```python
from build123d import *

# Parameters (mm, degrees)
EXTRUDE_THIN1_DEPTH = 10
FILLET1_R           = 5
FILLET2_R           = 5
FILLET3_R           = 5
FILLET4_R           = 5
FILLET5_R           = 5
CUT_EXTRUDE1_DEPTH  = 4.5


with BuildPart() as part:
    # Sketch1 → Extrude-Thin1 (new body)
    with BuildSketch(Plane.XY):
        with BuildLine():
            Line((5, 0), (5, 44.72135955))
            ThreePointArc((5, 44.72135955), (32.200514423, 31.434485377), (44.828761414, 3.922008424))
            Line((44.828761414, 3.922008424), (54.790708395, 4.793565851))
            ThreePointArc((54.790708395, 4.793565851), (35.273871656, 42.198980774), (-5, 54.772255751))
            Line((-5, 54.772255751), (-5, 0))
            Line((-5, 0), (5, 0))
        make_face()
    extrude(amount=EXTRUDE_THIN1_DEPTH)

    # Fillet1
    fillet1_edges = [part.edges().sort_by_distance(p)[0] for p in [
        (-5, 54.772255751, 5),
    ]]
    fillet(fillet1_edges, radius=FILLET1_R)

    # Fillet2
    fillet2_edges = [part.edges().sort_by_distance(p)[0] for p in [
        (54.790708395, 4.793565851, 5),
    ]]
    fillet(fillet2_edges, radius=FILLET2_R)

    # Fillet3
    fillet3_edges = [part.edges().sort_by_distance(p)[0] for p in [
        (44.828761414, 3.922008424, 5),
    ]]
    fillet(fillet3_edges, radius=FILLET3_R - 0.0001)  # a hair under: the kernel refuses the full size

    # Fillet4
    fillet4_edges = [part.edges().sort_by_distance(p)[0] for p in [
        (5, 0, 5),
    ]]
    fillet(fillet4_edges, radius=FILLET4_R)

    # Fillet5
    fillet5_edges = [part.edges().sort_by_distance(p)[0] for p in [
        (-5, 0, 5),
    ]]
    fillet(fillet5_edges, radius=FILLET5_R - 0.0001)  # a hair under: the kernel refuses the full size

    # Sketch2 → Cut-Extrude1 (cut)
    with BuildSketch(Plane(origin=(0, 0, 0), x_dir=(-1, 0, 0), z_dir=(0, 0, -1))):
        with BuildLine():
            Line((1.923996328, 19.347205988), (2.921, 7.13741415))
            ThreePointArc((2.921, 7.13741415), (0, 1.3805), (-2.921, 7.13741415))
            Line((-2.921, 7.13741415), (-1.923996328, 19.347205988))
            ThreePointArc((-1.923996328, 19.347205988), (0, 21.1205), (1.923996328, 19.347205988))
        make_face()
    extrude(amount=-CUT_EXTRUDE1_DEPTH, mode=Mode.SUBTRACT)


solid = part.part
```
Could you check a few things on this model? Use its own coordinates, in mm. A direction names the side the tool comes from. Round coordinates to 2 decimals unless told otherwise and drop trailing zeros. Write each loop counter-clockwise with the first axis right and the second up, starting at its lowest first coordinate (ties: lowest second). Pieces come first, ordered by that corner, then holes. Notation, with made-up numbers: M 41,62 L 54,62 A26 ccw 54,91 Z; hole C 11.5,73 d8. An arc over 180 degrees is marked long. Answer in a Markdown table with one row per item. Add a question column.
Q1. Imagine slicing it at B-B (y = 31.5). Please give me the cut outline in (x, z).
Q2. If we mould it in two halves opening along Y, with no side actions, what happens to faces 1 (the flat face through (-5, 28, 5)), 2 (the cylindrical face through (46.15, 5.3, 5.07)), 3 (the flat face through (0, 11, 4.5))? For each: +Y half, -Y half, draft (parallel to the pull), parting line (faces both ways), or undercut.
Q3. Will these pins go through, and if not, where does the flat tip stop? pin 1 Ø2 at (x, y) = (-1.5, 14) entering from -Z; pin 2 Ø5 at (y, z) = (14, 9) entering from +X.
Q4. Imagine slicing it at C-C (x = 45.5). Please give me the cut outline in (y, z).
Q5. On a 3-axis mill with a long thin cutter (end or side, diameter ignored), from which of +Z, -Z, +X, -X, +Y, -Y can I reach the whole of each face in a straight line? I mean faces 4 (the cylindrical face through (30.29, 33.28, 4.93)), 5 (the cylindrical face through (-0.112, 1.382, 2.218)), 6 (the cylindrical face through (35.489, 42.018, 4.93)). Say none if no direction works.
Q6. Imagine slicing it at D-D (x = 21). Please give me the cut outline in (y, z).
Q7. If I drill on line 1 (X direction, y = 5, z = 2.25); line 2 (X direction, y = 19.5, z = 4); line 3 (X direction, y = 34, z = 8.5), over which ranges is the centre line in solid material (lowest first)? Write a range as from..to.
Values:
| question | item | result |
|---|---|---|
| 1 | outline | M -5,0 L 5,0 L 5,10 L -5,10 Z; M 32.14,0 L 45.09,0 L 45.09,10 L 32.14,10 Z |
| 2 | face 1 | draft |
| 2 | face 2 | -Y half |
| 2 | face 3 | undercut |
| 3 | pin 1 | z = 0 |
| 3 | pin 2 | x = 53.78 |
| 4 | outline | M 5.87,0 L 30.9,0 L 30.9,10 L 5.87,10 Z |
| 5 | face 4 | +Z, -Z, -Y |
| 5 | face 5 | -Z |
| 5 | face 6 | +Z, -Z, +X, +Y |
| 6 | outline | M 39.8,0 L 50.83,0 L 50.83,10 L 39.8,10 Z |
| 7 | line 1 | -5..-3.62, 3.62..5, 46.6..51.65 |
| 7 | line 2 | -5..-1.91, 1.91..5, 40.56..51.43 |
| 7 | line 3 | -5..5, 29.48..43.23 |
